Source: CAD feature listing. Evaluate the final solid. Frame: model axes, mm. A direction names the side the tool comes from. Give positions to 0.01 mm unless a question says otherwise; leave off trailing zeros. Order: outer loops, then holes, each group sorted by start corner. A loop starts at its lowest first (then second) coordinate and runs counter-clockwise, first axis right, second up. Notation, with made-up numbers: M 57.5,8 L 72.5,8 A16 ccw 72.5,13 Z; hole C 12.25,15 d4. An arc over 180 degrees is marked long. Use CSV: the item, a comma, the result in double quotes. Start each with the question number.
Item 1: Section query B-B on x = 8. Count the separate pieces of the cut face and the enclosed holes in it, and give its area (3 significant figures).
Item 2: Section query D-D on x = -4.5. Return loops of the section in (y, z), and give its area (3 significant figures).
Item 3: Section query A-A on y = 6. Return loops of the section in (x, z).
Item 4: Pull-direction query (Y, two-part tool) for faces 3 (the face through (-10.05, 1.01, 5.91)), 4 (the face through (7.556, 11.999, 1.014)), 5 (the face through (3, 2, 14)); classes: +Y half, -Y half, draft (parallel to the pull), parting line (faces both ways), or undercut.
Item 5: First-contact query: pin 1 (6.5 mm diameter, centred on x = 0, y = 14, fed in from +Z); pin 2 (12 mm diameter, centred on x = 5, z = 17.5, fed in from +Y). Flat tips, straight axial feed; report the tip coordinate or a pass-through.
Item 6: Ray query, probe 1 along Z at (x, y) = (8, 1); probe 2 along X at (y, z) = (0.8, 22). Return the intervals inside material, ascending. Write a range as from..to.
Item 7: Access query for faces 1 (the face through (3, 0, 13)), 2 (the face through (0, 17, 2)). Directions: +Z, -Z, +X, -X, +Y, -Y. A direction counts if a zero-diameter tool reaches every point of the face in a straight line with its end or side. Return the directions, or none.
from build123d import *

# Parameters (mm, degrees)
BOSS_EXTRUDE1_DEPTH     = 12
SKETCH3_R               = 2.05
CUT_EXTRUDE1_DEPTH      = 25
CUT_EXTRUDE1_DEPTH_BACK = 3
SKETCH4_R               = 2.05
CUT_EXTRUDE2_DEPTH      = 3


with BuildPart() as part:
    # Sketch1 → Boss-Extrude1 (new body, symmetric)
    with BuildSketch(Plane(origin=(0, 0, 0), x_dir=(0, 0, -1), z_dir=(1, 0, 0))):
        Polygon((0, 0), (0, 26), (-2, 26), (-2, 2), (-26, 2), (-26, 0), align=None)
    extrude(amount=BOSS_EXTRUDE1_DEPTH, both=True)

    # Sketch3 → Cut-Extrude1 (cut, two sides)
    with BuildSketch(Plane.XY.offset(2)) as cut_extrude1_sk:
        with Locations((-8, 22)):
            Circle(SKETCH3_R)
        with Locations((0, 22)):
            Circle(SKETCH3_R)
        with Locations((8, 22)):
            Circle(SKETCH3_R)
        with Locations((0, 14)):
            Circle(SKETCH3_R)
        with Locations((8, 14)):
            Circle(SKETCH3_R)
        with Locations((0, 6)):
            Circle(SKETCH3_R)
        with Locations((8, 6)):
            Circle(SKETCH3_R)
        with Locations((-8, 14)):
            Circle(SKETCH3_R)
        with Locations((-8, 6)):
            Circle(SKETCH3_R)
    extrude(amount=CUT_EXTRUDE1_DEPTH, mode=Mode.SUBTRACT)
    extrude(cut_extrude1_sk.sketch, amount=-CUT_EXTRUDE1_DEPTH_BACK, mode=Mode.SUBTRACT)

    # Sketch4 → Cut-Extrude2 (cut, through all)
    with BuildSketch(Plane(origin=(0, 2, 0), x_dir=(1, 0, 0), z_dir=(0, 1, 0))):
        with Locations((-8, -22)):
            Circle(SKETCH4_R)
        with Locations((0, -22)):
            Circle(SKETCH4_R)
        with Locations((8, -22)):
            Circle(SKETCH4_R)
        with Locations((0, -14)):
            Circle(SKETCH4_R)
        with Locations((8, -14)):
            Circle(SKETCH4_R)
        with Locations((0, -6)):
            Circle(SKETCH4_R)
        with Locations((8, -6)):
            Circle(SKETCH4_R)
        with Locations((-8, -14)):
            Circle(SKETCH4_R)
        with Locations((-8, -6)):
            Circle(SKETCH4_R)
    extrude(amount=-CUT_EXTRUDE2_DEPTH, mode=Mode.SUBTRACT)


solid = part.part
Verdict:
1,separate pieces,"7"
1,enclosed holes,"0"
1,area,"50.8 mm2"
2,outline,"M 0,0 L 26,0 L 26,2 L 2,2 L 2,26 L 0,26 Z"
2,area,"100 mm2"
3,outline,"M -12,0 L -10.05,0 L -10.05,2 L -12,2 Z; M -5.95,0 L -2.05,0 L -2.05,2 L -5.95,2 Z; M 2.05,0 L 5.95,0 L 5.95,2 L 2.05,2 Z; M 10.05,0 L 12,0 L 12,2 L 10.05,2 Z"
4,face 3,"draft"
4,face 4,"undercut"
4,face 5,"+Y half"
5,pin 1,"z = 2"
5,pin 2,"y = 2"
6,probe 1,"0..3.95, 8.05..11.95, 16.05..19.95, 24.05..26"
6,probe 2,"-12..-10.05, -5.95..-2.05, 2.05..5.95, 10.05..12"
7,face 1,"+Z, -Z, +X, -X, -Y"
7,face 2,"+Z, +X, -X, +Y"
